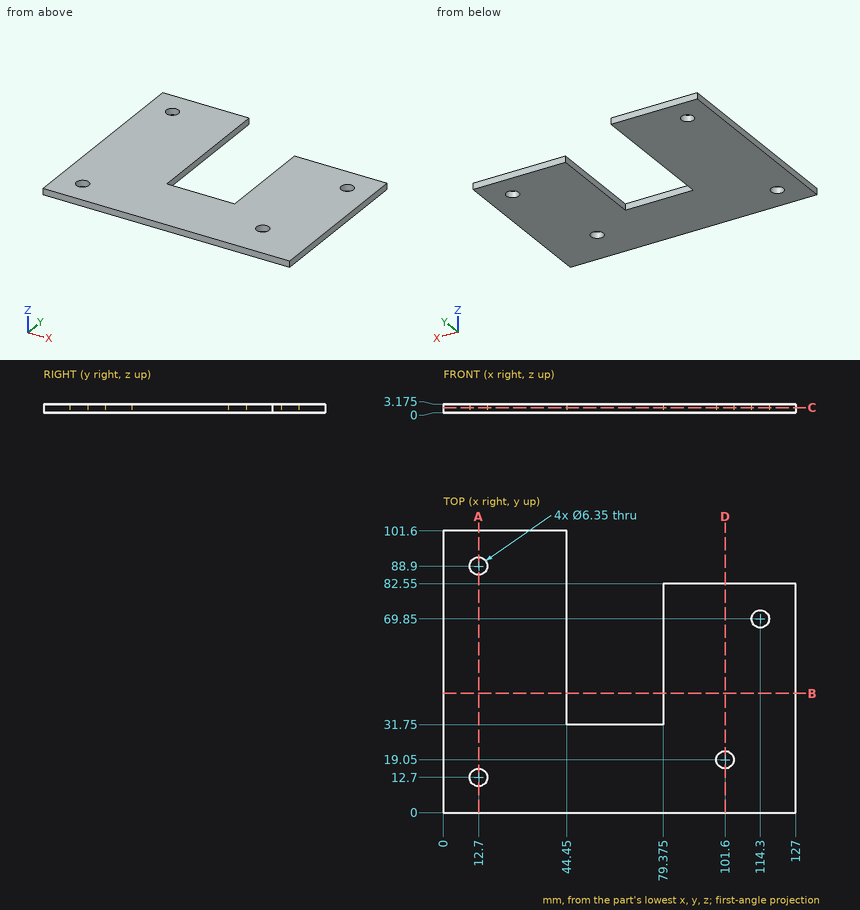
Here's the drawing with two shaded views (mm, measured from the low corner). I have some questions. Give positions to 0.01 mm unless a question says otherwise; leave off trailing zeros. Write each loop counter-clockwise with the first axis right and the second up, starting at its lowest first coordinate (ties: lowest second). Pieces come first, ordered by that corner, then holes. Notation, with made-up numbers: (75.5, -27.5) - (107.5, -27.5) arc R18 cw to (107.5, -9.5) - close; hole circle Ø1 at (54.25, 67). An arc over 180 degrees is marked (long way). One line per item, written item: value. Start each with the question number.
Item 1: Imagine slicing it at B-B, the plane y = 43. List the corners of the cut face in (x, z) for me (3 decimals), and give its area (3 significant figures).
Item 2: Imagine slicing it at C-C, the plane z = 1.85. List the corners of the cut face in (x, y) for me (3 decimals).
Item 3: Imagine slicing it at A-A, the plane x = 12.7. List the corners of the cut face in (y, z) for me (3 decimals).
Item 4: Please list where these lines run through material, in increasing order: line 1 (X direction, y = 69.85, z = 0.8) (3 decimals); line 2 (X direction, y = 12.7, z = 0.75) (3 decimals); line 3 (X direction, y = 82, z = 0.15) (3 decimals). Write a range as from..to.
Item 5: Imagine slicing it at D-D, the plane x = 101.6. List the corners of the cut face in (y, z) for me (3 decimals).
Geometry says:
1. outline: (0, 0) - (44.45, 0) - (44.45, 3.175) - (0, 3.175) - close; (79.375, 0) - (127, 0) - (127, 3.175) - (79.375, 3.175) - close
1. area: 292 mm^2
2. outline: (0, 0) - (127, 0) - (127, 82.55) - (79.375, 82.55) - (79.375, 31.75) - (44.45, 31.75) - (44.45, 101.6) - (0, 101.6) - close; hole circle Ø6.35 at (12.7, 12.7); hole circle Ø6.35 at (12.7, 88.9); hole circle Ø6.35 at (101.6, 19.05); hole circle Ø6.35 at (114.3, 69.85)
3. outline: (0, 0) - (9.525, 0) - (9.525, 3.175) - (0, 3.175) - close; (15.875, 0) - (85.725, 0) - (85.725, 3.175) - (15.875, 3.175) - close; (92.075, 0) - (101.6, 0) - (101.6, 3.175) - (92.075, 3.175) - close
4. line 1: 0..44.45, 79.375..111.125, 117.475..127
4. line 2: 0..9.525, 15.875..127
4. line 3: 0..44.45, 79.375..127
5. outline: (0, 0) - (15.875, 0) - (15.875, 3.175) - (0, 3.175) - close; (22.225, 0) - (82.55, 0) - (82.55, 3.175) - (22.225, 3.175) - close
